Design review of the part built by this model. Coordinates are the model's own, in mm. Round coordinates to 2 decimals unless told otherwise and drop trailing zeros. Order: outer loops, then holes, each group sorted by start corner. A loop starts at its lowest first (then second) coordinate and runs counter-clockwise, first axis right, second up. Notation, with made-up numbers: M -16.75,66 L 41.25,66 A11 ccw 41.25,80 Z; hole C 72.5,-6 d11. An arc over 180 degrees is marked long. Write each question's results on one line, items separated by ' | '. Start each with the question number.
Item 1: Clearance check with flat-ended pins moving along their axes: pin 1 (8 mm diameter, centred on y = 243, z = -187, fed in from -X); pin 2 (1.5 mm diameter, centred on x = 38, y = 349, fed in from +Z); pin 3 (10 mm diameter, centred on y = 207, z = -106.5, fed in from -X). State where each tip first meets the part, or that it passes through.
Item 2: Wall thickness on line 1 (X direction, y = 183, z = -123.5); line 2 (X direction, y = 84, z = -192); line 3 (Z direction, x = 27.5, y = 152): over which ranges is each line inside the solid? List them lowest first. Write a range as [from, to].
Item 3: Take a section at B-B, the plane x = 86.5. Write out the cut boundary in (y, z), plus the area to 3 significant figures.
Item 4: Take a section at A-A, the plane y = 60.5. Write out the cut boundary in (x, z), plus the area to 3 significant figures.
```python
from build123d import *

# Parameters (mm, degrees)
STOCK_ACRYLIC_DOOR_MASTER_1_START     = 163.456714755
STOCK_ACRYLIC_DOOR_MASTER_1_OUTLINE_W = 243.269145362
STOCK_ACRYLIC_DOOR_MASTER_1_OUTLINE_H = 433.75
STOCK_ACRYLIC_DOOR_MASTER_1_OUTLINE_R = 2
STOCK_ACRYLIC_DOOR_MASTER_1_DEPTH     = 5
SKETCH1_W                             = 0.25
SKETCH1_H                             = 433.75
CUT_EXTRUDE1_DEPTH                    = 438.771536387


# Read off the part's stored shape, not the designer's step: Stock-acrylic-door-master-1
with BuildPart() as part:
    # Stock-acrylic-door-master-1 outline → Stock-acrylic-door-master-1 (new body)
    with BuildSketch(Plane(origin=(0, 0, 0), x_dir=(0.866025403784438, 0, 0.500000000000001), z_dir=(0.500000000000001, 0, -0.866025403784438)).offset(STOCK_ACRYLIC_DOOR_MASTER_1_START)):
        with Locations((0, -202.375)):
            Rectangle(STOCK_ACRYLIC_DOOR_MASTER_1_OUTLINE_W, STOCK_ACRYLIC_DOOR_MASTER_1_OUTLINE_H)
        with Locations((-109.384572681, -389.875)):
            Circle(STOCK_ACRYLIC_DOOR_MASTER_1_OUTLINE_R, mode=Mode.SUBTRACT)
        with Locations((-109.384572681, -364.875)):
            Circle(STOCK_ACRYLIC_DOOR_MASTER_1_OUTLINE_R, mode=Mode.SUBTRACT)
        with Locations((-101.634572681, -242.375)):
            Circle(STOCK_ACRYLIC_DOOR_MASTER_1_OUTLINE_R, mode=Mode.SUBTRACT)
        with BuildLine():
            Line((108.884572681, -387.875), (109.884572681, -387.875))
            ThreePointArc((109.884572681, -387.875), (111.884572681, -389.875), (109.884572681, -391.875))
            Line((109.884572681, -391.875), (108.884572681, -391.875))
            ThreePointArc((108.884572681, -391.875), (106.884572681, -389.875), (108.884572681, -387.875))
        make_face(mode=Mode.SUBTRACT)
        with BuildLine():
            Line((108.884572681, -362.875), (109.884572681, -362.875))
            ThreePointArc((109.884572681, -362.875), (111.884572681, -364.875), (109.884572681, -366.875))
            Line((109.884572681, -366.875), (108.884572681, -366.875))
            ThreePointArc((108.884572681, -366.875), (106.884572681, -364.875), (108.884572681, -362.875))
        make_face(mode=Mode.SUBTRACT)
        with Locations((-101.634572681, -162.375)):
            Circle(STOCK_ACRYLIC_DOOR_MASTER_1_OUTLINE_R, mode=Mode.SUBTRACT)
        with Locations((-109.384572681, -39.875)):
            Circle(STOCK_ACRYLIC_DOOR_MASTER_1_OUTLINE_R, mode=Mode.SUBTRACT)
        with Locations((-109.384572681, -14.875)):
            Circle(STOCK_ACRYLIC_DOOR_MASTER_1_OUTLINE_R, mode=Mode.SUBTRACT)
        with BuildLine():
            Line((108.884572681, -37.875), (109.884572681, -37.875))
            ThreePointArc((109.884572681, -37.875), (111.884572681, -39.875), (109.884572681, -41.875))
            Line((109.884572681, -41.875), (108.884572681, -41.875))
            ThreePointArc((108.884572681, -41.875), (106.884572681, -39.875), (108.884572681, -37.875))
        make_face(mode=Mode.SUBTRACT)
        with BuildLine():
            Line((108.884572681, -12.875), (109.884572681, -12.875))
            ThreePointArc((109.884572681, -12.875), (111.884572681, -14.875), (109.884572681, -16.875))
            Line((109.884572681, -16.875), (108.884572681, -16.875))
            ThreePointArc((108.884572681, -16.875), (106.884572681, -14.875), (108.884572681, -12.875))
        make_face(mode=Mode.SUBTRACT)
    extrude(amount=STOCK_ACRYLIC_DOOR_MASTER_1_DEPTH)

    # Sketch1 → Cut-Extrude1 (cut, through all)
    with BuildSketch(Plane(origin=(84.228357378, 0, -145.887794416), x_dir=(-0.866025403784438, 0, -0.5000000000000012), z_dir=(0.5000000000000011, 0, -0.8660254037844379))):
        with Locations((-121.509572681, 202.375)):
            Rectangle(SKETCH1_W, SKETCH1_H)
        with Locations((121.509572681, 202.375)):
            Rectangle(SKETCH1_W, SKETCH1_H)
    extrude(amount=-CUT_EXTRUDE1_DEPTH, mode=Mode.SUBTRACT)


solid = part.part
```
Results list:
1) pin 1: x = -3.91 | pin 2: z = -166.37 | pin 3: x = 133.79
2) line 1: [113.01, 123.01] | line 2: [-5.64, 4.36] | line 3: [-178.64, -172.87]
3) outline: M -14.5,-144.58 L 419.25,-144.58 L 419.25,-138.8 L -14.5,-138.8 Z | area: 2,500 mm²
4) outline: M -23.39,-202.25 L -20.89,-206.58 L 189.35,-85.2 L 186.85,-80.87 Z | area: 1,210 mm²
